Verification items for the finished model (mm, model axes). A direction names the side the tool comes from. Coordinates: 2 decimals unless noted, no trailing zeros. Order: outer loops, then holes, each group sorted by start corner. A loop starts at its lowest first (then second) coordinate and runs counter-clockwise, first axis right, second up.
Q1. Draft check along Z on faces 1 (the cylindrical face through (-23.846, 2.028, 7.509)), 2 (the cylindrical face through (-24.124, 2.218, 0.049)), 3 (the flat face through (-11, 4, 23)). Enter one of: pulls with the +Z half, pulls with the -Z half, needs draft (parallel to the pull), parting line crosses it, or undercut.
Q2. Thickness scan on line 1 (Z direction, x = 0, y = 3.75); line 2 (X direction, y = 2.5, z = 1); line 3 (Z direction, x = -11, y = 2.25). Record the ranges inside material, lowest first.
Q3. Set-up check for faces 4 (the cylindrical face through (21.876, 2.218, 0.049)), 5 (the flat face through (22, 6, -2)): record each of +Z, -Z, +X, -X, +Y, -Y from which the full face is reachable in a straight line by a thin tool's end or side.
Q4. Cross-section at A-A, the plane z = 0. Record the boundary of the cut face in (x, y) (3 decimals).
Q5. Cross-section at B-B, the plane x = 0. Record the boundary of the cut face in (y, z).
Q6. Depth check by flat-ended pin: P1, Ø3, axis at x = 21.5, y = 3, coming from the +Z side; P2, Ø1.2, axis at x = 23, z = 0, coming from the +Y side; P3, Ø1.7, axis at x = 22, y = 6.5, coming from the +Z side; P4, Ø1, axis at x = -11.5, y = 1.5, coming from the +Z side. Enter the tip coordinate at first touch or a pass-through.
Q7. Cross-section at C-C, the plane y = 1.25. Record the boundary of the cut face in (x, z) (3 decimals).
from build123d import *

# Parameters (mm, degrees)
SKETCH2_R          = 1.125
CUT_EXTRUDE1_DEPTH = 8.5
CUT_EXTRUDE3_DEPTH = 3


with BuildPart() as part:
    # Sketch1 → Revolve1 (revolve)
    with BuildSketch(Plane.XY):
        Polygon((-29, 5), (-29, 6.5), (-28, 7.5), (-21, 7.5), (-21, 0), (-25, 0), (-25, 4), (-28, 4), align=None)
    revolve(axis=Axis((0, 0, 0), (0, 1, 0)))

    # Sketch2 → Cut-Extrude1 (cut, through all)
    with BuildSketch(Plane.XZ):
        with Locations((-23, 0)):
            Circle(SKETCH2_R)
        with Locations((23, 0)):
            Circle(SKETCH2_R)
    extrude(amount=-CUT_EXTRUDE1_DEPTH, mode=Mode.SUBTRACT)

    # Sketch3 → Cut-Extrude3 (cut)
    with BuildSketch(Plane(origin=(0, 7.5, 0), x_dir=(1, 0, 0), z_dir=(0, 1, 0))):
        with BuildLine():
            Line((-23, 2), (23, 2))
            ThreePointArc((23, 2), (25, 0), (23, -2))
            Line((23, -2), (-23, -2))
            ThreePointArc((-23, -2), (-25, 0), (-23, 2))
        make_face()
    extrude(amount=-CUT_EXTRUDE3_DEPTH, mode=Mode.SUBTRACT)


solid = part.part
Check values:
1. face 1: parting line crosses it
1. face 2: undercut
1. face 3: needs draft
2. line 1: z = -25 to -21, 21 to 25
2. line 2: x = -24.98 to -23.52, -22.48 to -20.98, 20.98 to 22.48, 23.52 to 24.98
2. line 3: z = -22.45 to -17.89, 17.89 to 22.45
3. face 4: +Y, -Y
3. face 5: +Y
4. outline: (-29, 5) - (-28, 4) - (-25, 4) - (-25, 0) - (-24.125, 0) - (-24.125, 4.5) - (-25, 4.5) - (-25, 7.5) - (-28, 7.5) - (-29, 6.5) - close; (-21.875, 0) - (-21, 0) - (-21, 4.5) - (-21.875, 4.5) - close; (21, 0) - (21.875, 0) - (21.875, 4.5) - (21, 4.5) - close; (24.125, 0) - (25, 0) - (25, 4) - (28, 4) - (29, 5) - (29, 6.5) - (28, 7.5) - (25, 7.5) - (25, 4.5) - (24.125, 4.5) - close
5. outline: (0, -25) - (4, -25) - (4, -28) - (5, -29) - (6.5, -29) - (7.5, -28) - (7.5, -21) - (0, -21) - close; (0, 21) - (7.5, 21) - (7.5, 28) - (6.5, 29) - (5, 29) - (4, 28) - (4, 25) - (0, 25) - close
6. P1: stops at z = 19.26
6. P2: passes through
6. P3: stops at z = 19.84
6. P4: stops at z = 22.45
7. outline: circle Ø50 at (0, 0); hole circle Ø2.25 at (-23, 0); hole circle Ø42 at (0, 0); hole circle Ø2.25 at (23, 0)
